Part model, mm, in its own coordinate system. Round coordinates to 2 decimals unless told otherwise and drop trailing zeros. Loops run counter-clockwise (first coordinate to the right, second up) from the corner with the lowest first, then second, coordinate; pieces in that order, holes last. Notation, with made-up numbers: (62.25, 23.5) -> (94.25, 23.5) arc R24 cw to (94.25, 56.5) -> close; hole circle Ø6 at (60.5, 49). An arc over 180 degrees is marked (long way). Use a Markdown table: item, result. Add a question column.
Item 1: Cut at B-B, the plane x = -21. List the corners of the cut face in (y, z), plus the area to 3 significant figures.
Item 2: Cut at A-A, the plane y = -5. List the corners of the cut face in (x, z).
Item 3: Probe line 1 (X direction, y = -5, z = 20); line 2 (Y direction, x = 21, z = 9.75); line 3 (X direction, y = -6.75, z = 3). List the from-to ranges inside material, lowest first. Write a range as [from, to].
Item 4: Flat gauge pins, fed straight in: pin 1 (1.5 mm diameter, centred on x = -2, y = -7, fed in from -Z); pin 2 (12 mm diameter, centred on x = 0.5, z = 18, fed in from +Y); pin 3 (5 mm diameter, centred on x = 2.5, y = -7.5, fed in from -Z). Where does each tip first touch, or does it go through?
Item 5: Two-plate mould, pull along Y, no slides. Class faces 1 (the face through (-16.836, -4.453, 12.675)), 2 (the face through (0, -5, 16)), 3 (the face through (0, 0, 18)): pulls with the +Y half, pulls with the -Y half, needs draft (parallel to the pull), parting line crosses it, or undercut.
Item 6: Cut at D-D, the plane z = 12.5. List the corners of the cut face in (x, y), plus the area to 3 significant figures.
Item 7: Cut at C-C, the plane z = 5.75. List the corners of the cut face in (x, y).
Solid Edge part; units mm, degrees
sketch "Sketch1" plane through (0, 0, 0) normal (0, -1, 0) x (1, 0, 0)
  line L0 (-26, 0) -> (-16, 0)
  arc A0 (-16, 0) -> (16, 0) centre (0, 0) cw
  line L1 (26, 0) -> (16, 0)
  line L2 (26, 25) -> (26, 0)
  line L3 (-26, 25) -> (26, 25)
  line L4 (-26, 0) -> (-26, 25)
  dimension "D1" = 26
  dimension "D2" = 26
extrude "Protrusion1" add sketch "Sketch1" along normal blind 10
hole "Hole_1" at (-21, -5, 25) direction (0, 0, -1) diameter 8.4 end up to next
hole "Hole1" at (21, -5, 25) direction (0, 0, -1) diameter 8.4 end up to next
properties material "Stainless Steel, 420"
A:
| question | item | result |
|---|---|---|
| 1 | outline | (-10, 0) -> (-9.2, 0) -> (-9.2, 25) -> (-10, 25) -> close; (-0.8, 0) -> (0, 0) -> (0, 25) -> (-0.8, 25) -> close |
| 1 | area | 40.0 mm^2 |
| 2 | outline | (-26, 0) -> (-25.2, 0) -> (-25.2, 25) -> (-26, 25) -> close; (-16.8, 0) -> (-16, 0) arc R16 cw to (16, 0) -> (16.8, 0) -> (16.8, 25) -> (-16.8, 25) -> close; (25.2, 0) -> (26, 0) -> (26, 25) -> (25.2, 25) -> close |
| 3 | line 1 | x = [-26, -25.2], [-16.8, 16.8], [25.2, 26] |
| 3 | line 2 | y = [-10, -9.2], [-0.8, 0] |
| 3 | line 3 | x = [-26, -24.82], [-17.18, -15.72], [15.72, 17.18], [24.82, 26] |
| 4 | pin 1 | stops at z = 15.76 |
| 4 | pin 2 | stops at y = 0 |
| 4 | pin 3 | stops at z = 15.2 |
| 5 | face 1 | undercut |
| 5 | face 2 | needs draft |
| 5 | face 3 | pulls with the +Y half |
| 6 | outline | (-26, -10) -> (-9.99, -10) -> (-9.99, 0) -> (-26, 0) -> close; (9.99, -10) -> (26, -10) -> (26, 0) -> (9.99, 0) -> close; hole circle Ø8.4 at (-21, -5); hole circle Ø8.4 at (21, -5) |
| 6 | area | 209 mm^2 |
| 7 | outline | (-26, -10) -> (-14.93, -10) -> (-14.93, 0) -> (-26, 0) -> close; (14.93, -10) -> (26, -10) -> (26, 0) -> (14.93, 0) -> close; hole circle Ø8.4 at (-21, -5); hole circle Ø8.4 at (21, -5) |
